```python
from build123d import *

# Parameters (mm, degrees)
SKETCH_1_W                  = 595
SKETCH_1_H                  = 38
EXTRUDE_1_DEPTH             = 5
HOLE_WIZARD_M3_1_D          = 2.5
PATTERN_LINEAR_1_COUNT      = 12
PATTERN_LINEAR_1_PITCH      = 50
SKETCH_4_W                  = 595
SKETCH_4_H                  = 12
CUT_EXTRUDE_1_DEPTH         = 1
SKETCH_5_W                  = 5
SKETCH_5_H                  = 38
EXTRUDE_2_DEPTH             = 8
HOLE_WIZARD_M4_1_D          = 3.3
HOLE_WIZARD_M4_1_DEPTH      = 6
HOLE_WIZARD_M4_1_TIP        = 0.991420021
EXTRUDE_3_DEPTH             = 10
HOLE_WIZARD_M4_2_D          = 3.3
HOLE_WIZARD_M4_2_DEPTH      = 10.1
HOLE_WIZARD_M4_2_TIP        = 0.991420021
HOLE_WIZARD_M3_2_AT_2_COUNT = 2
HOLE_WIZARD_M3_2_AT_2_PITCH = 19
PATTERN_LINEAR_2_COUNT      = 2
PATTERN_LINEAR_2_PITCH      = 120
PATTERN_LINEAR_3_COUNT      = 2
PATTERN_LINEAR_3_PITCH      = 430
EXTRUDE_4_DEPTH             = 50
EXTRUDE_5_DEPTH             = 50
SKETCH_18_R                 = 2.75
CUT_EXTRUDE_2_DEPTH         = 8
SKETCH_19_R                 = 2.75
CUT_EXTRUDE_3_DEPTH         = 8
SKETCH_20_R                 = 2.75
CUT_EXTRUDE_4_DEPTH         = 8


with BuildPart() as part:
    # 草图1 → 凸台-拉伸1 (new body)
    with BuildSketch(Plane.XY):
        with Locations((297.5, 19)):
            Rectangle(SKETCH_1_W, SKETCH_1_H)
    extrude(amount=EXTRUDE_1_DEPTH)

    # M3 螺纹孔1 (through all)
    with Locations(Plane.XY.offset(5)):
        with Locations((10, 19)):
            hole_wizard_m3_1 = Hole(HOLE_WIZARD_M3_1_D / 2)

    # 阵列(线性)1: M3 螺纹孔1 ×12
    with Locations(*[(i * PATTERN_LINEAR_1_PITCH, 0, 0) for i in range(1, PATTERN_LINEAR_1_COUNT)]):
        add(hole_wizard_m3_1, mode=Mode.SUBTRACT)

    # 草图4 → 切除-拉伸1 (cut)
    with BuildSketch(Plane.XY.offset(5)):
        with Locations((297.5, 19)):
            Rectangle(SKETCH_4_W, SKETCH_4_H)
    extrude(amount=-CUT_EXTRUDE_1_DEPTH, mode=Mode.SUBTRACT)

    # 草图5 → 凸台-拉伸2 (add)
    with BuildSketch(Plane.ZY):
        with Locations((-2.5, 19)):
            Rectangle(SKETCH_5_W, SKETCH_5_H)
    extrude(amount=-EXTRUDE_2_DEPTH)

    # M4 螺纹孔1
    with Locations(Plane.ZY):
        with Locations((0.69552528, 14), (0.69552528, 4)):
            Hole(HOLE_WIZARD_M4_1_D / 2, depth=HOLE_WIZARD_M4_1_DEPTH)
            with Locations((0, 0, -(HOLE_WIZARD_M4_1_DEPTH + HOLE_WIZARD_M4_1_TIP / 2))):  # 118° drill point
                Cone(0, HOLE_WIZARD_M4_1_D / 2, HOLE_WIZARD_M4_1_TIP, mode=Mode.SUBTRACT)

    # 草图8 → 凸台-拉伸3 (add)
    with BuildSketch(Plane(origin=(595, 0, 0), x_dir=(0, 0, -1), z_dir=(1, 0, 0))):
        Polygon((-5, 0), (-5, 13), (-4, 13), (-4, 25), (-5, 25), (-5, 38), (0, 38), (0, 0), align=None)
    extrude(amount=EXTRUDE_3_DEPTH)

    # M4 螺纹孔2
    with Locations(Plane.XY.offset(5)):
        with Locations((598.5, 9.00237217), (590.5, 9.00237217)):
            Hole(HOLE_WIZARD_M4_2_D / 2, depth=HOLE_WIZARD_M4_2_DEPTH)
            with Locations((0, 0, -(HOLE_WIZARD_M4_2_DEPTH + HOLE_WIZARD_M4_2_TIP / 2))):  # 118° drill point
                Cone(0, HOLE_WIZARD_M4_2_D / 2, HOLE_WIZARD_M4_2_TIP, mode=Mode.SUBTRACT)

    # 草图13 → M3 螺纹孔2 (revolve, cut)
    with BuildSketch(Plane(origin=(44.992811473, 31.7, 0), x_dir=(0, 1, 0), z_dir=(1, 0, 0))):
        Polygon((0, 0), (0, 8.251075774), (1.25, 7.5), (1.25, 0), align=None)
    hole_wizard_m3_2 = revolve(axis=Axis((44.992811473, 31.7, -6.35), (0, 0, 1)), mode=Mode.SUBTRACT)

    # M3 螺纹孔2 at 2: M3 螺纹孔2 ×2
    with Locations(*[(i * HOLE_WIZARD_M3_2_AT_2_PITCH, 0, 0) for i in range(1, HOLE_WIZARD_M3_2_AT_2_COUNT)]):
        add(hole_wizard_m3_2, mode=Mode.SUBTRACT)

    # 阵列(线性)2: M3 螺纹孔2 ×2
    with Locations(*[(i * PATTERN_LINEAR_2_PITCH, 0, 0) for i in range(1, PATTERN_LINEAR_2_COUNT)]):
        add(hole_wizard_m3_2, mode=Mode.SUBTRACT)

    # 阵列(线性)2 copy 1 sketch → 阵列(线性)2 copy 1 (revolve, cut)
    with BuildSketch(Plane(origin=(183.992811473, 31.7, 0), x_dir=(0, 1, 0), z_dir=(1, 0, 0))):
        Polygon((0, 0), (0, 8.251075774), (1.25, 7.5), (1.25, 0), align=None)
    revolve(axis=Axis((183.992811473, 31.7, -6.35), (0, 0, 1)), mode=Mode.SUBTRACT)

    # 阵列(线性)3: M3 螺纹孔2 ×2
    with Locations(*[(i * PATTERN_LINEAR_3_PITCH, 0, 0) for i in range(1, PATTERN_LINEAR_3_COUNT)]):
        add(hole_wizard_m3_2, mode=Mode.SUBTRACT)

    # 阵列(线性)3 copy 1 sketch → 阵列(线性)3 copy 1 (revolve, cut)
    with BuildSketch(Plane(origin=(493.992811473, 31.7, 0), x_dir=(0, 1, 0), z_dir=(1, 0, 0))):
        Polygon((0, 0), (0, 8.251075774), (1.25, 7.5), (1.25, 0), align=None)
    revolve(axis=Axis((493.992811473, 31.7, -6.35), (0, 0, 1)), mode=Mode.SUBTRACT)

    # 草图14 → 凸台-拉伸4 (add)
    with BuildSketch(Plane.XZ):
        Polygon((8, -5), (0, -5), (0, 5), (30, 5), (30, 0), (8, 0), align=None)
    extrude(amount=EXTRUDE_4_DEPTH)

    # 草图15 → 凸台-拉伸5 (add)
    with BuildSketch(Plane(origin=(0, 38, 0), x_dir=(1, 0, 0), z_dir=(0, 1, 0))):
        Polygon((0, 5), (0, -5), (30, -5), (30, 0), (8, 0), (8, 5), align=None)
    extrude(amount=EXTRUDE_5_DEPTH)

    # 草图18 → 切除-拉伸2 (cut)
    with BuildSketch(Plane.XY.offset(5)):
        with Locations((25, 73)):
            Circle(SKETCH_18_R)
        with Locations((13, 73)):
            Circle(SKETCH_18_R)
        with Locations((13, -35)):
            Circle(SKETCH_18_R)
        with Locations((25, -35)):
            Circle(SKETCH_18_R)
    extrude(amount=-CUT_EXTRUDE_2_DEPTH, mode=Mode.SUBTRACT)

    # 草图19 → 切除-拉伸3 (cut)
    with BuildSketch(Plane.XY.offset(5)):
        with Locations((585, 31.5)):
            Circle(SKETCH_19_R)
        with Locations((597, 31.5)):
            Circle(SKETCH_19_R)
    extrude(amount=-CUT_EXTRUDE_3_DEPTH, mode=Mode.SUBTRACT)

    # 草图20 → 切除-拉伸4 (cut)
    with BuildSketch(Plane.XY.offset(5)):
        with Locations((235.288610816, 31.5)):
            Circle(SKETCH_20_R)
        with Locations((223.288610816, 31.5)):
            Circle(SKETCH_20_R)
    extrude(amount=-CUT_EXTRUDE_4_DEPTH, mode=Mode.SUBTRACT)


solid = part.part
```
Design review of the part built by this model. Coordinates are the model's own, in mm. A direction names the side the tool comes from. Round coordinates to 2 decimals unless told otherwise and drop trailing zeros. Write each loop counter-clockwise with the first axis right and the second up, starting at its lowest first coordinate (ties: lowest second). Pieces come first, ordered by that corner, then holes. Notation, with made-up numbers: (8.5, -29.5) -> (22.5, -29.5) arc R25 ccw to (22.5, 5.5) -> close; hole circle Ø5 at (43, 85). An arc over 180 degrees is marked (long way). Answer in a Markdown table with one row per item.
Q1. Draft analysis for pull direction Y (two halves, no side actions). For faces 1 (the face through (12, -50, 1)), 2 (the face through (298, 19, 4)), 3 (the face through (0, 18, 0)), state which applies: +Y half, -Y half, draft (parallel to the pull), parting line (faces both ways), or undercut.
The answers:
| item | result |
|---|---|
| face 1 | -Y half |
| face 2 | undercut |
| face 3 | draft |
Q2. Take a section at A-A, the plane y = 60.5. State the section outline as (x, z) points, then the cut area to 3 significant figures.
The answers:
| item | result |
|---|---|
| outline | (0, -5) -> (8, -5) -> (8, 0) -> (30, 0) -> (30, 5) -> (0, 5) -> close |
| area | 190 mm² |
Q3. Clearance check with flat-ended pins moving along their axes: pin 1 Ø6 at (x, z) = (209, -2.5) entering from -Y; pin 2 Ø2 at (x, y) = (164.99, 31.7) entering from -Z; pin 3 Ø4 at (y, z) = (39, -3.5) entering from +X; pin 4 Ø2.5 at (x, z) = (203.5, 2.5) entering from +Y. State where each tip first meets the part, or that it passes through.
The answers:
| item | result |
|---|---|
| pin 1 | y = 0 |
| pin 2 | through |
| pin 3 | x = 8 |
| pin 4 | y = 38 |
Q4. For faces 4 (the face through (256, 35, 5)), 5 (the face through (286, 14, 0)), list the 3-axis set-ups (+Z, -Z, +X, -X, +Y, -Y) from which the entire face can be reached by the end or side of a thin tool; tool diameter is ignored.
The answers:
| item | result |
|---|---|
| face 4 | +Z, +X, -X, +Y, -Y |
| face 5 | -Z, +X, +Y, -Y |
Q5. Take a section at B-B, the plane z = -2.5. State the section outline as (x, y) points.
The answers:
| item | result |
|---|---|
| outline | (0, -50) -> (8, -50) -> (8, 88) -> (0, 88) -> close |
Q6. To check wall thickness, follow L1, parallel to Y at x = 460, z = 2.9; L2, parallel to X at y = 9, z = 1.5; L3, parallel to Y at x = 25, z = 2.05. State the ranges of each line that lie inside material, in increasing order. Write a range as [from, to].
The answers:
| item | result |
|---|---|
| L1 | [0, 17.75], [20.25, 38] |
| L2 | [0, 588.85], [592.15, 596.85], [600.15, 605] |
| L3 | [-50, -37.75], [-32.25, 70.25], [75.75, 88] |
